Input: part model. Units: mm. Frame: model coordinates. Face numbers are marked on the shaded views. A direction names the side the tool comes from. Give positions to 0.01 mm unless a question says otherwise; leave off trailing zeros. Loops run counter-clockwise (first coordinate to the right, second up) from the corner with the lowest first, then second, coordinate; pieces in that order, holes last. Notation, with made-up numbers: M 13.25,-8.75 L 40.25,-8.75 A26 ccw 40.25,9.25 Z; hole C -40,-35.75 d2. An arc over 180 degrees is marked long. Return JSON: item names as keys, results as strings. Group by question number.
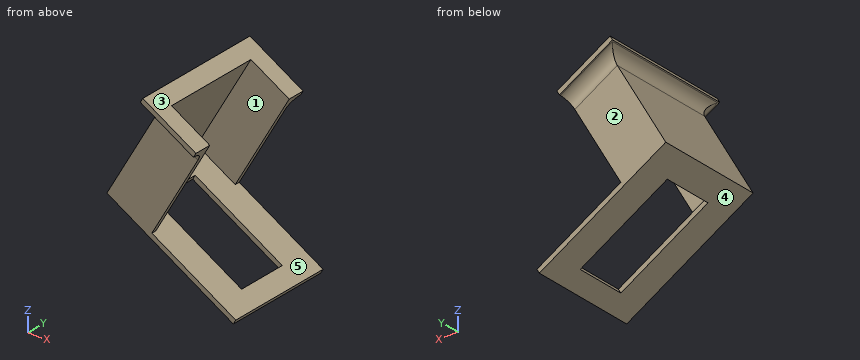
```python
from build123d import *

# Parameters (mm, degrees)
SKETCH029_W             = 59.5
SKETCH029_H             = 44
SKETCH029_W_2           = 41
SKETCH029_H_2           = 20.5
PAD015_DEPTH            = 2
PAD016_DEPTH            = 44
PAD017_DEPTH            = 2
FILLET_R                = 4.5
BODY011_PLACEMENT_ANGLE = 210


with BuildPart() as part:
    # Sketch029 → Pad015 (new body)
    with BuildSketch(Plane.XY):
        with Locations((1.25, 0.25)):
            Rectangle(SKETCH029_W, SKETCH029_H)
        Rectangle(SKETCH029_W_2, SKETCH029_H_2, mode=Mode.SUBTRACT)
    extrude(amount=PAD015_DEPTH)

    # Sketch030 (on Face9 of Pad015) → Pad016 (join)
    with BuildSketch(Plane(origin=(0, 0, 0), x_dir=(1, 0, 0), z_dir=(0, 0, -1))):
        Polygon((31, 21.75), (31, -22.25), (11, -22.25), (11, -20.25), (29, -20.25), (29, 19.75), (11, 19.75), (11, 21.75), align=None)
    extrude(amount=PAD016_DEPTH)

    # Sketch031 (on Face18 of Pad016) → Pad017 (join)
    with BuildSketch(Plane(origin=(0, 0, -44), x_dir=(1, 0, 0), z_dir=(0, 0, -1))):
        Polygon((11, 19.75), (11, 26.75), (36, 26.75), (36, -27.25), (11, -27.25), (11, -20.25), (29, -20.25), (29, 19.75), align=None)
    extrude(amount=-PAD017_DEPTH)

    # Fillet
    fillet_edges = [part.edges().sort_by_distance(p)[0] for p in [
        (31, 0.25, -42),
        (21, 22.25, -42),
        (21, -21.75, -42),
    ]]
    fillet(fillet_edges, radius=FILLET_R)


with BuildPart() as part_1:
    # Body011 placement: moved
    add(part.part.moved(Location((-6.411543, 0, -47.105118))).rotate(Axis((-6.411543, 0, -47.105118), (0, 1, 0)), BODY011_PLACEMENT_ANGLE))


solid = part_1.part
```
Item 1: Section C-C, the plane z = -39.5. Return loops of the section in (x, y).
Item 2: Pull-direction query (Y, two-part tool) for the marked faces 1, 2 and 3; classes: pulls with the +Y half, pulls with the -Y half, needs draft (parallel to the pull), parting line crosses it, or undercut.
Item 3: Section A-A, the plane y = 3.5. Return loops of the section in (x, z), then the cut area to 3 significant figures.
Item 4: Section B-B, the plane x = 7. Return loops of the section in (y, z), then the cut area to 3 significant figures.
Item 5: Material intervals for line 1 (Y direction, x = -24, z = -28.5); line 2 (Y direction, x = 0.5, z = -1); line 3 (Z direction, x = -16, y = -11), sorted ascending. Write a range as from..to.
Item 6: First-contact query: pin 1 Ø1 at (x, y) = (-17.5, 2) entering from -Z; pin 2 Ø11 at (x, z) = (-11, -43.5) entering from +Y; pin 3 Ø19 at (x, z) = (-19.5, -21) entering from -Y. Flat tips, straight axial feed; report the tip coordinate or a pass-through.
Item 7: Reachability of the marked faces 4 and 5 from +Z, -Z, +X, -X, +Y, -Y: full face, straight path, thin tool, end or side. Return the list, or none.
Item 8: Section D-D, the plane y = 12. Return loops of the section in (x, z), then the cut area to 3 significant figures.
Answer below:
{
 "1": {"outline": "M -23.58,-21.75 L -14.72,-21.75 L -14.72,-19.75 L -19.58,-19.75 L -19.58,-10.25 L -23.58,-10.25 Z; M -23.58,10.25 L -19.58,10.25 L -19.58,20.25 L -14.72,20.25 L -14.72,22.25 L -23.58,22.25 Z"},
 "2": {"face 1": "undercut", "face 2": "pulls with the +Y half", "face 3": "needs draft"},
 "3": {"outline": "M -34.26,-33.34 L -25.17,-38.59 L -24.17,-36.86 L -31.53,-32.61 L -9.53,5.5 L -15.59,9 L -16.59,7.27 L -16.16,7.02 A4.5 cw -14.51,0.87 Z; M 10.34,-59.09 L 17.27,-63.09 L 18.27,-61.36 L 11.34,-57.36 Z", "area": "139 mm^2"},
 "4": {"outline": "M -21.75,-57.16 L -10.25,-57.16 L -10.25,-54.85 L -21.75,-54.85 Z; M 10.25,-57.16 L 22.25,-57.16 L 22.25,-54.85 L 10.25,-54.85 Z", "area": "54.3 mm^2"},
 "5": {"line 1": "-21.75..-19.75, 20.25..22.25", "line 2": "-26.75..-19.75, 20.25..27.25", "line 3": "-43.88..-41.57, -5.71..-1.71, 6.92..8.29"},
 "6": {"pin 1": "z = -9.18", "pin 2": "y = 22.25", "pin 3": "y = -21.75"},
 "7": {"face 4": "-Z, -X, +Y, -Y", "face 5": "+X"},
 "8": {"outline": "M -34.26,-33.34 L 17.27,-63.09 L 18.27,-61.36 L -31.53,-32.61 L -9.53,5.5 L -15.59,9 L -16.59,7.27 L -16.16,7.02 A4.5 cw -14.51,0.87 Z", "area": "221 mm^2"}
}
